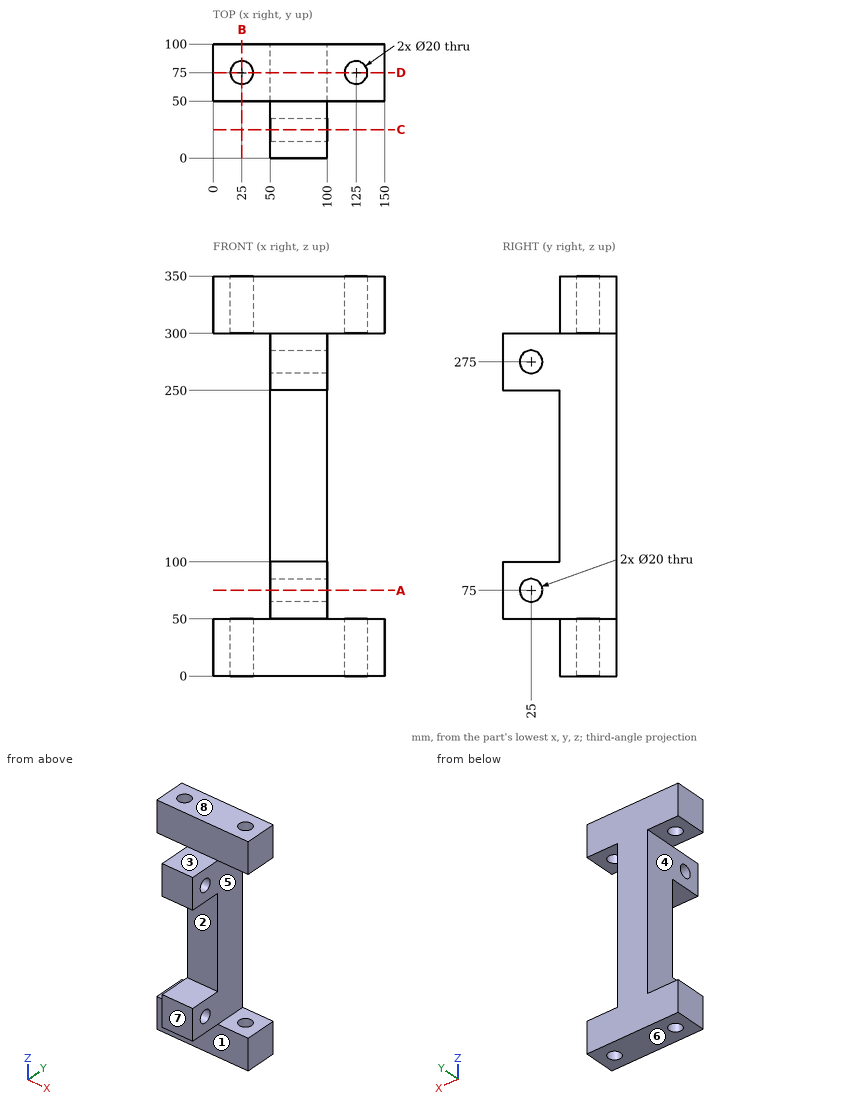
Design review of the part shown in the three views and the two pictorial views. Dimensions are in mm from the part's minimum x, y and z. A direction names the side the tool comes from. Round coordinates to 2 decimals unless told otherwise and drop trailing zeros. Order: outer loops, then holes, each group sorted by start corner. A loop starts at its lowest first (then second) coordinate and runs counter-clockwise, first axis right, second up. Notation, with made-up numbers: M 22.25,37.25 L 66.25,37.25 A19 cw 66.25,65.25 Z; hole C 13.5,-6 d9. An arc over 180 degrees is marked long. Put each result on its own line as item: value.
Q1. Consider section A-A (z = 75). State the section outline as (x, y) points, and give its area (3 significant figures).
Reported:
outline: M 50,0 L 100,0 L 100,15 L 50,15 Z; M 50,35 L 100,35 L 100,100 L 50,100 Z
area: 4,000 mm²
Q2. Consider section D-D (y = 75). State the section outline as (x, z) points.
Reported:
outline: M 0,0 L 15,0 L 15,50 L 0,50 Z; M 0,300 L 15,300 L 15,350 L 0,350 Z; M 35,0 L 115,0 L 115,50 L 100,50 L 100,300 L 115,300 L 115,350 L 35,350 L 35,300 L 50,300 L 50,50 L 35,50 Z; M 135,0 L 150,0 L 150,50 L 135,50 Z; M 135,300 L 150,300 L 150,350 L 135,350 Z
Q3. Consider section C-C (y = 25). State the section outline as (x, z) points.
Reported:
outline: M 50,50 L 100,50 L 100,65 L 50,65 Z; M 50,85 L 100,85 L 100,100 L 50,100 Z; M 50,250 L 100,250 L 100,265 L 50,265 Z; M 50,285 L 100,285 L 100,300 L 50,300 Z
Q4. Draft analysis for pull direction Z (two halves, no side actions). For the marked faces 5, 6, 7 and 8, state which applies: released by +Z, released by -Z, zero draft, split by the parting line, or undercut.
Reported:
face 5: undercut
face 6: released by -Z
face 7: zero draft
face 8: released by +Z
Q5. To check wall thickness, follow line 1 (Z direction, x = 66.5, y = 26); line 2 (Y direction, x = 125, z = 12); line 3 (X direction, y = 67, z = 334). State the ranges of each line that lie inside material, in increasing order.
Reported:
line 1: 50 to 65.05, 84.95 to 100, 250 to 265.05, 284.95 to 300
line 2: 50 to 65, 85 to 100
line 3: 0 to 19, 31 to 119, 131 to 150
Q6. Insertion check: pin 1 Ø18 at (x, y) = (25, 75) entering from +Z; pin 2 Ø1 at (y, z) = (17, 252) entering from -X; pin 3 Ø15 at (x, y) = (85, 19.5) entering from -Z; pin 4 Ø15 at (x, y) = (80, 27) entering from +Z. Each pin has a flat end and moves straight along its axis. Give the tip position at first contact, or say it passes through.
Reported:
pin 1: through
pin 2: x = 50
pin 3: z = 50
pin 4: z = 300
Q7. Machinability: for the marked faces 1, 2, 3 and 4, which of the approach directions +Z, -Z, +X, -X, +Y, -Y give a long, thin tool a straight path to every point of the face, cutting with its end or side? Answer none if there is none.
Reported:
face 1: -Z, +X, -X, -Y
face 2: +X, -X, -Y
face 3: +Z, +X, -X, -Y
face 4: -X, +Y, -Y
Q8. Consider section B-B (x = 25). State the section outline as (y, z) points, and give its area (3 significant figures).
Reported:
outline: M 50,0 L 65,0 L 65,50 L 50,50 Z; M 50,300 L 65,300 L 65,350 L 50,350 Z; M 85,0 L 100,0 L 100,50 L 85,50 Z; M 85,300 L 100,300 L 100,350 L 85,350 Z
area: 3,000 mm²
